Can you work these out from the model? Positions are in its coordinate system, mm. A direction names the side the tool comes from. Coordinates: 2 decimals unless noted, no trailing zeros. Order: outer loops, then holes, each group sorted by start corner. A loop starts at its lowest first (then second) coordinate and runs counter-clockwise, first axis right, second up. Notation, with made-up numbers: (63.25, 13) -> (95.25, 13) arc R31 ccw to (95.25, 45) -> close; hole circle Ø3 at (50, 16.25). An arc over 180 degrees is marked (long way). Use a Markdown table: item, result. Add a question column.
1. For faces 1 (the cylindrical face through (-98.67, 24.74, 1.23)), 2 (the cylindrical face through (-82.49, 1.41, 1.23)), 3 (the flat face through (-109, 17.3, -10)), 4 (the flat face through (-96, 11, 0)), 5 (the flat face through (-109, -0.95, 1)), which set-ups out of +Z, -Z, +X, -X, +Y, -Y let a thin tool reach every point of the face, with its end or its side?
2. Suppose I cut it at B-B, the plane x = -109.5. List the corners of the cut face in (y, z) for me.
3. For pin 1 Ø4 at (x, z) = (-115.5, -9) entering from +Y; pin 2 Ø3 at (x, y) = (-96.5, 11.5) entering from +Z; pin 3 Ø2 at (y, z) = (12.5, -10) entering from +X, each with a flat end and sliding along its axis, tell me the tip position at first contact or that it passes through.
4. Suppose I cut it at A-A, the plane y = 11.8. State how many separate pieces and enclosed holes the cut face has, then the cut area to 3 significant figures.
5. If I drill on line 1 along X through (y, z) = (11.8, -5.75); line 2 along X through (y, z) = (11.8, -9.75); line 3 along Z through (x, y) = (-124.5, -0.5), over which ranges is the centre line in solid material (lowest first)? Write a range as from..to.
6. Suppose I cut it at D-D, the plane z = -7.75. List the corners of the cut face in (x, y) for me, then the cut area to 3 significant figures.
7. We'd pull the mould along Y, two halves only. Please class faces 6 (the flat face through (-95.85, -4.19, 1.23)), 7 (the cylindrical face through (-136.578, 24.877, 1.232)), 8 (the cylindrical face through (-127.65, 11.96, -1.05)): pulls with the +Y half, pulls with the -Y half, needs draft (parallel to the pull), parting line crosses it, or undercut.
8. Suppose I cut it at C-C, the plane z = -1. List the corners of the cut face in (x, y) for me, then the cut area to 3 significant figures.
```python
from build123d import *

# Parameters (mm, degrees)
SKETCH1_RX              = 2
SKETCH1_RY              = 2
BOSS_EXTRUDE1_DEPTH     = 2.5
SKETCH14_W              = 31.891524792
SKETCH14_H              = 10.99995058
BOSS_EXTRUDE9_DEPTH     = 13.5
CUT_EXTRUDE2_DEPTH      = 142.15856284
CUT_EXTRUDE2_DEPTH_BACK = 142.15856284
SKETCH12_R              = 1.25
FILLET9_R               = 6
SKETCH15_R              = 2.75
SKETCH15_R_2            = 3
CUT_EXTRUDE3_DEPTH      = 2.5


with BuildPart() as part:
    # Sketch1 → Boss-Extrude1 (new body)
    with BuildSketch(Plane.XY):
        with BuildLine():
            Line((-97.997023968, -1.656563984), (-93.647036265, -6.786872031))
            ThreePointArc((-93.647036265, -6.786872031), (-91.040064157, -8.175287806), (-88.191031172, -7.396177424))
            Line((-88.191031172, -7.396177424), (-82.596119502, -3.186067977))
            ThreePointArc((-82.596119502, -3.186067977), (-81.610744956, -1.2458696), (-82.196119502, 0.85))
            ThreePointArc((-82.196119502, 0.85), (-82.493486098, 1.417544468), (-82.596119502, 2.05))
            Line((-82.596119502, 2.05), (-82.596119502, 21.55))
            ThreePointArc((-82.596119502, 21.55), (-82.493486098, 22.182455532), (-82.196119502, 22.75))
            ThreePointArc((-82.196119502, 22.75), (-81.610744956, 24.8458696), (-82.596119502, 26.786067977))
            Line((-82.596119502, 26.786067977), (-88.191031172, 30.996177424))
            ThreePointArc((-88.191031172, 30.996177424), (-91.040064157, 31.775287806), (-93.647036265, 30.386872031))
            Line((-93.647036265, 30.386872031), (-97.997023968, 25.256563984))
            ThreePointArc((-97.997023968, 25.256563984), (-98.681908745, 24.735217364), (-99.522482349, 24.55))
            Line((-99.522482349, 24.55), (-118.669756656, 24.55))
            ThreePointArc((-118.669756656, 24.55), (-119.51033026, 24.735217364), (-120.195215037, 25.256563984))
            Line((-120.195215037, 25.256563984), (-124.54520274, 30.386872031))
            ThreePointArc((-124.54520274, 30.386872031), (-127.152174848, 31.775287806), (-130.001207832, 30.996177424))
            Line((-130.001207832, 30.996177424), (-135.596119502, 26.786067977))
            ThreePointArc((-135.596119502, 26.786067977), (-136.581494048, 24.8458696), (-135.996119502, 22.75))
            ThreePointArc((-135.996119502, 22.75), (-135.698752906, 22.182455532), (-135.596119502, 21.55))
            Line((-135.596119502, 21.55), (-135.596119502, 2.05))
            ThreePointArc((-135.596119502, 2.05), (-135.698752906, 1.417544468), (-135.996119502, 0.85))
            ThreePointArc((-135.996119502, 0.85), (-136.581494048, -1.2458696), (-135.596119502, -3.186067977))
            Line((-135.596119502, -3.186067977), (-130.001207832, -7.396177424))
            ThreePointArc((-130.001207832, -7.396177424), (-127.152174848, -8.175287806), (-124.54520274, -6.786872031))
            Line((-124.54520274, -6.786872031), (-120.195215037, -1.656563984))
            ThreePointArc((-120.195215037, -1.656563984), (-119.51033026, -1.135217364), (-118.669756656, -0.95))
            Line((-118.669756656, -0.95), (-99.522482349, -0.95))
            ThreePointArc((-99.522482349, -0.95), (-98.681908745, -1.135217364), (-97.997023968, -1.656563984))
        make_face()
        with Locations(Location((-90.596119502, 27.8), (0, 0, 61.223751036))):
            Ellipse(SKETCH1_RX, SKETCH1_RY, mode=Mode.SUBTRACT)
        with Locations(Location((-127.596119502, 27.8), (0, 0, -118.776248964))):
            Ellipse(SKETCH1_RX, SKETCH1_RY, mode=Mode.SUBTRACT)
        with Locations(Location((-127.596119502, -4.2), (0, 0, -118.776248964))):
            Ellipse(SKETCH1_RX, SKETCH1_RY, mode=Mode.SUBTRACT)
        with Locations(Location((-90.596119502, -4.2), (0, 0, -28.776248964))):
            Ellipse(SKETCH1_RX, SKETCH1_RY, mode=Mode.SUBTRACT)
    extrude(amount=BOSS_EXTRUDE1_DEPTH)

    # Sketch14 → Boss-Extrude9 (add)
    with BuildSketch(Plane(origin=(0, 0, 0), x_dir=(-1, 0, 0), z_dir=(0, 0, -1))):
        with Locations((109.096119502, 11.8)):
            Rectangle(SKETCH14_W, SKETCH14_H)
    extrude(amount=BOSS_EXTRUDE9_DEPTH)

    # Sketch12 → Cut-Extrude2 (cut, two sides: drawn at the far end of the back side and taken through both)
    with BuildSketch(Plane.XY.offset(2.5).offset(-CUT_EXTRUDE2_DEPTH_BACK)):
        with Locations((-97.596119502, 11.8)):
            Circle(SKETCH12_R)
        with Locations((-120.596119502, 11.8)):
            Circle(SKETCH12_R)
        with Locations((-109.096119502, 11.8)):
            Circle(SKETCH12_R)
    extrude(amount=CUT_EXTRUDE2_DEPTH + CUT_EXTRUDE2_DEPTH_BACK, mode=Mode.SUBTRACT)

    # Fillet9
    fillet9_edges = [part.edges().sort_by_distance(p)[0] for p in [
        (-93.150357106, 11.8, 0),
        (-109.096119502, 6.30002471, 0),
        (-125.041881898, 11.8, 0),
        (-109.096119502, 17.29997529, 0),
    ]]
    fillet(fillet9_edges, radius=FILLET9_R)

    # Sketch15 → Cut-Extrude3 (cut)
    with BuildSketch(Plane.XY.offset(2.5)):
        with Locations((-120.596119502, 11.8)):
            Circle(SKETCH15_R)
        with Locations((-109.096119502, 11.8)):
            Circle(SKETCH15_R_2)
        with Locations((-97.596119502, 11.8)):
            Circle(SKETCH15_R)
    extrude(amount=-CUT_EXTRUDE3_DEPTH, mode=Mode.SUBTRACT)


solid = part.part
```
Worked out:
| question | item | result |
|---|---|---|
| 1 | face 1 | +Z, -Z, +Y |
| 1 | face 2 | +Z, -Z, +X |
| 1 | face 3 | -Z, +X, -X, +Y |
| 1 | face 4 | +Z |
| 1 | face 5 | +Z, -Z, -Y |
| 2 | outline | (-0.95, 0) -> (0.3, 0) arc R6 cw to (6.3, -6) -> (6.3, -13.5) -> (10.62, -13.5) -> (10.62, 0) -> (8.83, 0) -> (8.83, 2.5) -> (-0.95, 2.5) -> close; (12.98, -13.5) -> (17.3, -13.5) -> (17.3, -6) arc R6 cw to (23.3, 0) -> (24.55, 0) -> (24.55, 2.5) -> (14.77, 2.5) -> (14.77, 0) -> (12.98, 0) -> close |
| 3 | pin 1 | stops at y = 17.3 |
| 3 | pin 2 | stops at z = 0 |
| 3 | pin 3 | stops at x = -93.15 |
| 4 | separate pieces | 4 |
| 4 | enclosed holes | 0 |
| 4 | area | 435 mm² |
| 5 | line 1 | x = -125.05..-121.85, -119.35..-110.35, -107.85..-98.85, -96.35..-93.15 |
| 5 | line 2 | x = -125.04..-121.85, -119.35..-110.35, -107.85..-98.85, -96.35..-93.15 |
| 5 | line 3 | z = 0..2.5 |
| 6 | outline | (-125.04, 6.3) -> (-93.15, 6.3) -> (-93.15, 17.3) -> (-125.04, 17.3) -> close; hole circle Ø2.5 at (-120.6, 11.8); hole circle Ø2.5 at (-109.1, 11.8); hole circle Ø2.5 at (-97.6, 11.8) |
| 6 | area | 336 mm² |
| 7 | face 6 | pulls with the -Y half |
| 7 | face 7 | undercut |
| 7 | face 8 | needs draft |
| 8 | outline | (-127.73, 3.62) -> (-90.47, 3.62) -> (-90.47, 19.98) -> (-127.73, 19.98) -> close; hole circle Ø2.5 at (-120.6, 11.8); hole circle Ø2.5 at (-109.1, 11.8); hole circle Ø2.5 at (-97.6, 11.8) |
| 8 | area | 595 mm² |
